from build123d import *

# Parameters (mm, degrees)
ESBO_O1_W                  = 50
ESBO_O1_H                  = 50
ESBO_O1_W_2                = 47
ESBO_O1_H_2                = 47
RESSALTO_EXTRUS_O1_DEPTH   = 50
ESBO_O3_R                  = 5
CORTE_EXTRUS_O1_DEPTH      = 1
CORTE_EXTRUS_O1_DEPTH_BACK = 51
ESBO_O2_R                  = 2.5
CORTE_EXTRUS_O2_DEPTH      = 10
ESBO_O5_R                  = 1.5
CORTE_EXTRUS_O3_DEPTH      = 1
CORTE_EXTRUS_O3_DEPTH_BACK = 51


with BuildPart() as part:
    # Esboço1 → Ressalto-extrusão1 (new body)
    with BuildSketch(Plane.XY):
        Rectangle(ESBO_O1_W, ESBO_O1_H)
        Rectangle(ESBO_O1_W_2, ESBO_O1_H_2, mode=Mode.SUBTRACT)
    extrude(amount=RESSALTO_EXTRUS_O1_DEPTH)

    # Esboço3 → Corte-extrusão1 (cut, two sides)
    with BuildSketch(Plane(origin=(25, 0, 0), x_dir=(0, 0, -1), z_dir=(1, 0, 0))) as corte_extrus_o1_sk:
        with Locations((-25, 0)):
            Circle(ESBO_O3_R)
    extrude(amount=CORTE_EXTRUS_O1_DEPTH, mode=Mode.SUBTRACT)
    extrude(corte_extrus_o1_sk.sketch, amount=-CORTE_EXTRUS_O1_DEPTH_BACK, mode=Mode.SUBTRACT)

    # Esboço2 → Corte-extrusão2 (cut)
    with BuildSketch(Plane(origin=(0, 25, 0), x_dir=(1, 0, 0), z_dir=(0, 1, 0))):
        with Locations((-8.838834765, -16.161165235)):
            Circle(ESBO_O2_R)
        with Locations((8.838834765, -16.161165235)):
            Circle(ESBO_O2_R)
        with Locations((-8.838834765, -33.838834765)):
            Circle(ESBO_O2_R)
        with Locations((8.838834765, -33.838834765)):
            Circle(ESBO_O2_R)
    extrude(amount=-CORTE_EXTRUS_O2_DEPTH, mode=Mode.SUBTRACT)

    # Esboço5 → Corte-extrusão3 (cut, two sides)
    with BuildSketch(Plane(origin=(25, 0, 0), x_dir=(0, 0, -1), z_dir=(1, 0, 0))) as corte_extrus_o3_sk:
        with Locations((-11.25, 0)):
            Circle(ESBO_O5_R)
        with Locations((-38.75, 0)):
            Circle(ESBO_O5_R)
    extrude(amount=CORTE_EXTRUS_O3_DEPTH, mode=Mode.SUBTRACT)
    extrude(corte_extrus_o3_sk.sketch, amount=-CORTE_EXTRUS_O3_DEPTH_BACK, mode=Mode.SUBTRACT)


solid = part.part
Geometry: final body of the model. Coordinates: model frame, mm. A direction names the side the tool comes from. Give positions to 0.01 mm unless a question says otherwise; leave off trailing zeros. Loops run counter-clockwise (first coordinate to the right, second up) from the corner with the lowest first, then second, coordinate; pieces in that order, holes last. Notation, with made-up numbers: M -36.5,10.5 L -14.5,10.5 A12 cw -14.5,22.5 Z; hole C -23.5,41.25 d5. An arc over 180 degrees is marked long. Put each result on its own line as item: value.
1) First-contact query: P1, Ø10, axis at x = 0.5, y = 19.5, coming from the -Z side; P2, Ø4, axis at x = -8.84, z = 33.84, coming from the +Y side; P3, Ø9, axis at y = 0, z = 25, coming from the +X side. Flat tips, straight axial feed; report the tip coordinate or a pass-through.
Computed values:
P1: stops at z = 0
P2: stops at y = -23.5
P3: passes through
2) Material intervals for L1, parallel to Y at x = 23, z = 38; L2, parallel to Y at x = -24.05, z = 38.75, sorted ascending. Write a range as from..to.
Computed values:
L1: y = -25..-23.5, 23.5..25
L2: y = -25..-1.5, 1.5..25
3) Cut plane B-B, the plane y = 18. Return the cut outline in (x, z).
Computed values:
outline: M -25,0 L -23.5,0 L -23.5,50 L -25,50 Z; M 23.5,0 L 25,0 L 25,50 L 23.5,50 Z
4) Reachability of faces 4 (the flat face through (23.5, -6, 25)), 5 (the cylindrical face through (24, 0, 30)), 6 (the cylindrical face through (10.18, 24.26, 31.73)) from +Z, -Z, +X, -X, +Y, -Y: full face, straight path, thin tool, end or side. Return the list, or none.
Computed values:
face 4: +Z, -Z
face 5: +X, -X
face 6: +Y
5) Mould query, pull axis Y, two halves, no side actions, for faces 1 (the cylindrical face through (-24.24, -0.91, 39.94)), 2 (the flat face through (-25, 0, 19)), 3 (the flat face through (0, -23.5, 25)). Classes: released by +Y, released by -Y, zero draft, split by the parting line, or undercut.
Computed values:
face 1: undercut
face 2: zero draft
face 3: undercut
6) Cut plane A-A, the plane z = 38.75. Return the cut outline in (x, y), plus the area to 3 significant figures.
Computed values:
outline: M -25,-25 L 25,-25 L 25,-1.5 L 23.5,-1.5 L 23.5,-23.5 L -23.5,-23.5 L -23.5,-1.5 L -25,-1.5 Z; M -25,1.5 L -23.5,1.5 L -23.5,23.5 L 23.5,23.5 L 23.5,1.5 L 25,1.5 L 25,25 L -25,25 Z
area: 282 mm^2
7) Cut plane D-D, the plane y = 0. Give the number of separate pieces and of enclosed holes in the cut face, plus the area to 3 significant figures.
Computed values:
separate pieces: 8
enclosed holes: 0
area: 102 mm^2
